Part model, mm, in its own coordinate system. A direction names the side the tool comes from. Give positions to 0.01 mm unless a question says otherwise; leave off trailing zeros. Write each loop counter-clockwise with the first axis right and the second up, starting at its lowest first coordinate (ties: lowest second). Pieces come first, ordered by that corner, then holes. Notation, with made-up numbers: M 51.25,-16.75 L 104.25,-16.75 A22 ccw 104.25,21.25 Z; hole C -22.5,55.25 d1. An arc over 180 degrees is marked long. Use a Markdown table: item, result. Add a question column.
from build123d import *

# Parameters (mm, degrees)
SKETCH1_W           = 30
SKETCH1_H           = 30
BOSS_EXTRUDE3_DEPTH = 10
SKETCH2_W           = 20
SKETCH2_H           = 10
BOSS_EXTRUDE5_DEPTH = 30
FILLET1_R           = 10
SKETCH8_R           = 4.75
CUT_EXTRUDE6_DEPTH  = 47.904157598
FILLET3_R           = 5


with BuildPart() as part:
    # Sketch1 → Boss-Extrude3 (new body)
    with BuildSketch(Plane.XY):
        with Locations((15, 15)):
            Rectangle(SKETCH1_W, SKETCH1_H)
    extrude(amount=BOSS_EXTRUDE3_DEPTH)

    # Sketch2 → Boss-Extrude5 (add)
    with BuildSketch(Plane.ZY):
        with Locations((20, 25)):
            Rectangle(SKETCH2_W, SKETCH2_H)
    extrude(amount=-BOSS_EXTRUDE5_DEPTH)

    # Fillet1
    fillet1_edges = [part.edges().sort_by_distance(p)[0] for p in [
        (15, 20, 10),
    ]]
    fillet(fillet1_edges, radius=FILLET1_R)

    # Sketch8 → Cut-Extrude6 (cut, through all)
    with BuildSketch(Plane.XZ.offset(-20)):
        with Locations(Location((15, 25, 0), (0, 0, 270))):
            Circle(SKETCH8_R)
    extrude(amount=-CUT_EXTRUDE6_DEPTH, mode=Mode.SUBTRACT)

    # Fillet3
    fillet3_edges = [part.edges().sort_by_distance(p)[0] for p in [
        (15, 30, 0),
    ]]
    fillet(fillet3_edges, radius=FILLET3_R)


solid = part.part
1. Cut at A-A (z = 25). Write the cut outline in (x, y).
2. Flat gauge pins, fed straight in: pin 1 (8 mm diameter, centred on x = 16.5, y = 2.5, fed in from +Z); pin 2 (3 mm diameter, centred on x = 16, z = 26, fed in from -Y); pin 3 (8 mm diameter, centred on x = 19, z = 22, fed in from -Y); pin 4 (10 mm diameter, centred on x = 3.5, y = 9.5, fed in from +Z). Where does each tip first touch, or does it go through?
3. Drill centre lines: probe 1 along X at (y, z) = (27, 25); probe 2 along Y at (x, z) = (9.75, 20.5); probe 3 along X at (y, z) = (25.5, 26.75). Where is each one in solid material? Low to high. Write a range as [from, to].
4. Cut at C-C (x = 23.5). Write the cut outline in (y, z).
5. Tool access for faces 5 (the flat face through (11, 20, 22)), 6 (the flat face through (15, 30, 17)): list every direction of +Z, -Z, +X, -X, +Y, -Y with a clear straight run to the whole face (end or side of a thin tool).
6. Mould opens along X. For faces 1 (the flat face through (30, 19, 11)), 2 (the cylindrical face through (13.181, 24.93, 20.612)), 3 (the flat face through (0, 19, 11)), 4 (the flat face through (15, 13, 0)) say: released by +X, released by -X, zero draft, split by the parting line, or undercut.
7. Cut at D-D (y = 18). Write the cut outline in (x, z), then the cut area to 3 significant figures.
8. Cut at B-B (x = 15). Write the cut outline in (y, z), then the cut area to 3 significant figures.
A:
| question | item | result |
|---|---|---|
| 1 | outline | M 0,20 L 10.25,20 L 10.25,30 L 0,30 Z; M 19.75,20 L 30,20 L 30,30 L 19.75,30 Z |
| 2 | pin 1 | stops at z = 10 |
| 2 | pin 2 | passes through |
| 2 | pin 3 | stops at y = 19.8 |
| 2 | pin 4 | stops at z = 11.07 |
| 3 | probe 1 | x = [0, 10.25], [19.75, 30] |
| 3 | probe 2 | y = [20, 30] |
| 3 | probe 3 | x = [0, 10.58], [19.42, 30] |
| 4 | outline | M 0,0 L 25,0 A5 ccw 30,5 L 30,30 L 20,30 L 20,20 A10 cw 10,10 L 0,10 Z |
| 5 | face 5 | +Z, +X, -X, -Y |
| 5 | face 6 | +Z, -Z, +X, -X, +Y |
| 6 | face 1 | released by +X |
| 6 | face 2 | undercut |
| 6 | face 3 | released by -X |
| 6 | face 4 | zero draft |
| 7 | outline | M 0,0 L 30,0 L 30,14 L 0,14 Z |
| 7 | area | 420 mm² |
| 8 | outline | M 0,0 L 25,0 A5 ccw 30,5 L 30,20.25 L 20,20.25 L 20,20 A10 cw 10,10 L 0,10 Z; M 20,29.75 L 30,29.75 L 30,30 L 20,30 Z |
| 8 | area | 421 mm² |
